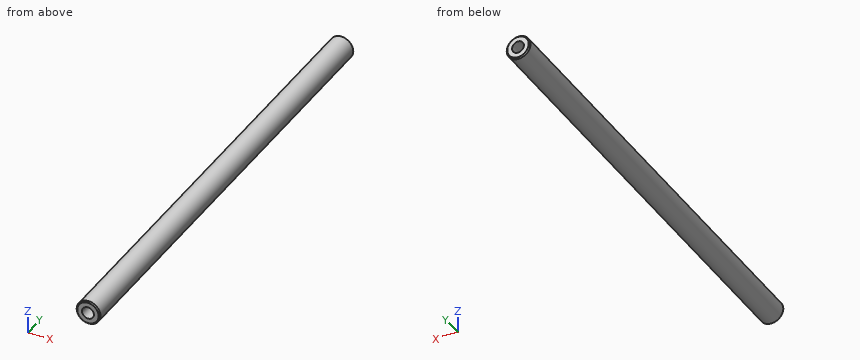
from build123d import *

# Parameters (mm, degrees)
ESQUISSE1_R      = 5
EXTRUSION1_DEPTH = 200
CHANFREIN1_SIZE  = 0.5
ESQUISSE2_R      = 2.5
EXTRUSION2_DEPTH = 15
ESQUISSE3_R      = 2.5
EXTRUSION3_DEPTH = 15


with BuildPart() as part:
    # Esquisse1 → Extrusion1 (new body)
    with BuildSketch(Plane(origin=(0, 0, 0), x_dir=(1, 0, 0), z_dir=(0, 1, 0))):
        Circle(ESQUISSE1_R)
    extrude(amount=EXTRUSION1_DEPTH)

    # Chanfrein1
    chanfrein1_edges = [part.edges().sort_by_distance(p)[0] for p in [
        (-5, 0, 0),
        (-5, 200, 0),
    ]]
    chamfer(chanfrein1_edges, length=CHANFREIN1_SIZE)

    # Esquisse2 → Extrusion2 (cut)
    with BuildSketch(Plane.XZ):
        Circle(ESQUISSE2_R)
    extrude(amount=-EXTRUSION2_DEPTH, mode=Mode.SUBTRACT)

    # Esquisse3 → Extrusion3 (cut)
    with BuildSketch(Plane(origin=(0, 200, 0), x_dir=(1, 0, 0), z_dir=(0, 1, 0))):
        Circle(ESQUISSE3_R)
    extrude(amount=-EXTRUSION3_DEPTH, mode=Mode.SUBTRACT)


solid = part.part
Verification items for the finished model (mm, model axes). Coordinates: 2 decimals unless noted, no trailing zeros. Write each loop counter-clockwise with the first axis right and the second up, starting at its lowest first coordinate (ties: lowest second). Pieces come first, ordered by that corner, then holes. Notation, with made-up numbers: (62.25, 28.5) -> (101.25, 28.5) arc R18 cw to (101.25, 44.5) -> close; hole circle Ø10 at (38, 63.25). An arc over 180 degrees is marked (long way). One line per item, written item: value. Start each with the question number.
Q1. Go/stop test with flat-tipped pins: P1, Ø1, axis at x = -3.5, y = 66, coming from the -Z side; P2, Ø3, axis at y = 73, z = 3.5, coming from the +X side; P3, Ø4, axis at y = 110, z = -3, coming from the -X side. Record where each tip stops, or that it passes through.
Q2. Cross-section at B-B on x = 0. Enter the section's corners in (y, z), and give its area (3 significant figures).
Q3. Thickness scan on L1, parallel to X at y = 196, z = 0; L2, parallel to Y at x = -0.75, z = 0.5. Record the ranges inside material, lowest first. Write a range as from..to.
Q4. Cross-section at C-C on y = 83. Enter the section's corners in (x, z).
Q5. Cross-section at A-A on z = 0. Enter the section's corners in (x, y), and give its area (3 significant figures).
Checked values:
1. P1: stops at z = -4
1. P2: stops at x = 4.58
1. P3: stops at x = -4.9
2. outline: (0, -4.5) -> (0.5, -5) -> (199.5, -5) -> (200, -4.5) -> (200, -2.5) -> (185, -2.5) -> (185, 2.5) -> (200, 2.5) -> (200, 4.5) -> (199.5, 5) -> (0.5, 5) -> (0, 4.5) -> (0, 2.5) -> (15, 2.5) -> (15, -2.5) -> (0, -2.5) -> close
2. area: 1,850 mm²
3. L1: x = -5..-2.5, 2.5..5
3. L2: y = 15..185
4. outline: circle Ø10 at (0, 0)
5. outline: (-5, 0.5) -> (-4.5, 0) -> (-2.5, 0) -> (-2.5, 15) -> (2.5, 15) -> (2.5, 0) -> (4.5, 0) -> (5, 0.5) -> (5, 199.5) -> (4.5, 200) -> (2.5, 200) -> (2.5, 185) -> (-2.5, 185) -> (-2.5, 200) -> (-4.5, 200) -> (-5, 199.5) -> close
5. area: 1,850 mm²
